Verification items for the finished model (mm, model axes). A direction names the side the tool comes from. Coordinates: 2 decimals unless noted, no trailing zeros. Loops run counter-clockwise (first coordinate to the right, second up) from the corner with the lowest first, then second, coordinate; pieces in that order, holes last.
Q1. Go/stop test with flat-tipped pins: P1, Ø0.6, axis at y = -6, z = -17, coming from the +X side; P2, Ø0.6, axis at x = -5, y = -4, coming from the +Z side; P3, Ø12, axis at x = -4.5, z = 2, coming from the -Y side. Record where each tip stops, or that it passes through.
Q2. Sectioned sample at C-C (x = -9.5). Enter the section's corners in (y, z).
Q3. Sectioned sample at A-A (z = 22). Enter the section's corners in (x, y), then the cut area to 3 significant figures.
Q4. Material ranges on probe 1 along Z at (x, y) = (0, -2.65); probe 2 along Z at (x, y) = (0, -3.95); probe 3 along Y at (x, z) = (-7.5, 17.5), recorded low to high.
Q5. Access from +Z, -Z, +X, -X, +Y, -Y to the whole of each face (thin tool, end or side, straight path). Record for faces 1 (the face through (3.374, -4.06, -1.503)), 2 (the face through (-8.597, -2.88, 27.073)).
Q6. Sectioned sample at B-B (z = -14). Enter the section's corners in (x, y), then the cut area to 3 significant figures.
Q7. Mould release check, pull along Z, two halves, no side actions. Record for faces 3 (the face through (0, -6.35, -15)), 4 (the face through (-9.165, -4.06, 5.715)), 5 (the face through (24.17, -2.88, 2.02)): +Z half, -Z half, draft (parallel to the pull), parting line (faces both ways), or undercut.
Q8. Sectioned sample at D-D (z = 14). Enter the section's corners in (x, y), then the cut area to 3 significant figures.
```python
from build123d import *

# Parameters (mm, degrees)
F0_R     = 1.182239
F0_R_2   = 0.817997
F1_DEPTH = 5.842
F2_DEPTH = 3.81
F3_DEPTH = 5.08
F4_DEPTH = 4.318
F5_R     = 1.71122
F6_DEPTH = 25.4
F7_DEPTH = 6.35


with BuildPart() as f1:
    # F0 (on Front) → F1 (new body)
    with BuildSketch(Plane.XZ):
        Polygon((-4.180855, -20.625193), (-4.353608, -20.920252), (-3.424949, -21.167446), (-3.28061, -20.625193), align=None)
        Polygon((3.424949, -21.167446), (4.353608, -20.920252), (4.180855, -20.625193), (3.28061, -20.625193), align=None)
        Polygon((22.26289, -6.835999), (22.26289, 1.657223), (4.394875, -5.754956), (2.197438, -5.957079), (0, -6.159202), (-2.197438, -5.957079), (-4.394875, -5.754956), (-22.26289, 1.657223), (-22.26289, -6.835999), (-22.832444, -9.118818), (-15.86828, -11.246894), (-14.217053, -15.145346), (-4.353608, -20.920252), (-4.180855, -20.625193), (-4.180855, -11.195441), (-3.601368, -9.465247), (0, -9.465247), (3.601368, -9.465247), (4.180855, -11.195441), (4.180855, -20.625193), (4.353608, -20.920252), (14.217053, -15.145346), (15.86828, -11.246894), (22.832444, -9.118818), align=None)
        Polygon((-15.86828, -11.246894), (-22.832444, -9.118818), (-22.26289, -10.434624), (-14.217053, -15.145346), align=None)
        Polygon((22.26289, -10.434624), (22.832444, -9.118818), (15.86828, -11.246894), (14.217053, -15.145346), align=None)
        Polygon((24.816887, 1.657223), (22.26289, 1.657223), (22.26289, -6.835999), (22.832444, -9.118818), (25.498668, -5.754956), align=None)
        with Locations((23.784082, -3.675047)):
            Circle(F0_R, mode=Mode.SUBTRACT)
        with Locations((23.597831, -0.42893)):
            Circle(F0_R_2, mode=Mode.SUBTRACT)
        Polygon((-22.26289, -6.835999), (-22.26289, 1.657223), (-24.816887, 1.657223), (-25.498668, -5.754956), (-22.832444, -9.118818), align=None)
        with Locations((-23.784082, -3.675047)):
            Circle(F0_R, mode=Mode.SUBTRACT)
        with Locations((-23.597831, -0.42893)):
            Circle(F0_R_2, mode=Mode.SUBTRACT)
        Polygon((-19.404403, 16.750786), (-22.26289, 15.816627), (-23.496922, 2.400486), (-22.26289, 1.657223), align=None)
        Polygon((23.496922, 2.400486), (22.26289, 15.816627), (19.404403, 16.750786), (22.26289, 1.657223), align=None)
        Polygon((24.816887, 1.657223), (23.496922, 2.400486), (22.26289, 1.657223), align=None)
        Polygon((-22.26289, 1.657223), (-23.496922, 2.400486), (-24.816887, 1.657223), align=None)
        Polygon((-19.404403, 16.750786), (-22.832444, 16.386179), (-22.26289, 15.816627), align=None)
        Polygon((22.26289, 15.816627), (22.832444, 16.386179), (19.404403, 16.750786), align=None)
        Polygon((22.832444, 16.386179), (22.136323, 20.879321), (5.009265, 22.700958), (2.695112, 21.684956), (0, 21.684956), (-2.695112, 21.684956), (-5.009265, 22.700958), (-22.136323, 20.879321), (-22.832444, 16.386179), (-19.404403, 16.750786), (-5.009265, 18.281856), (-2.695112, 17.265854), (0, 17.265854), (2.695112, 17.265854), (5.009265, 18.281856), (19.404403, 16.750786), align=None)
        Polygon((3.467637, 26.608711), (0, 26.608711), (-3.467637, 26.608711), (-4.353608, 27.524108), (-12.96019, 26.608711), (-16.187659, 24.61306), (-16.630644, 23.537237), (-22.136323, 20.879321), (-5.009265, 22.700958), (-2.695112, 21.684956), (0, 21.684956), (2.695112, 21.684956), (5.009265, 22.700958), (22.136323, 20.879321), (16.630644, 23.537237), (16.187659, 24.61306), (12.96019, 26.608711), (4.353608, 27.524108), align=None)
    extrude(amount=F1_DEPTH)

    # F0 (on Front) → F2 (join)
    with BuildSketch(Plane.XZ):
        with Locations((23.784082, -3.675047)):
            Circle(F0_R)
        with Locations((23.597831, -0.42893)):
            Circle(F0_R_2)
        with Locations((-23.784082, -3.675047)):
            Circle(F0_R)
        with Locations((-23.597831, -0.42893)):
            Circle(F0_R_2)
        Polygon((22.26289, 1.657223), (19.404403, 16.750786), (18.012892, 15.012917), (13.572707, 15.012917), (11.013955, 13.131482), (5.896451, 13.131482), (4.394875, 15.088174), (0, 15.088174), (-4.394875, 15.088174), (-5.896451, 13.131482), (-11.013955, 13.131482), (-13.572707, 15.012917), (-18.012892, 15.012917), (-19.404403, 16.750786), (-22.26289, 1.657223), (-4.394875, -5.754956), (-2.197438, -5.957079), (-1.331172, -3.868833), (0, -3.868833), (1.331172, -3.868833), (2.197438, -5.957079), (4.394875, -5.754956), align=None)
        Polygon((-2.750259, 0), (-4.015016, -3.048861), (-11.364689, 0), (-11.364689, 3.272761), (-7.025312, 8.089235), (-4.015016, 8.089235), (-1.832551, 11.701591), (0, 11.701591), (1.832551, 11.701591), (4.015016, 8.089235), (7.025312, 8.089235), (11.364689, 3.272761), (11.364689, 0), (4.015016, -3.048861), (2.750259, 0), (0, 0), align=None, mode=Mode.SUBTRACT)
    extrude(amount=F2_DEPTH)

    # F0 (on Front) → F3 (join)
    with BuildSketch(Plane.XZ):
        Polygon((0, -6.159202), (2.197438, -5.957079), (1.331172, -3.868833), (0, -3.868833), (-1.331172, -3.868833), (-2.197438, -5.957079), align=None)
    extrude(amount=F3_DEPTH)

    # F0 (on Front) → F4 (join)
    with BuildSketch(Plane.XZ):
        Polygon((-11.364689, 0), (-4.015016, -3.048861), (-2.750259, 0), (0, 0), (2.750259, 0), (4.015016, -3.048861), (11.364689, 0), (11.364689, 3.272761), (7.025312, 8.089235), (4.015016, 8.089235), (1.832551, 11.701591), (0, 11.701591), (-1.832551, 11.701591), (-4.015016, 8.089235), (-7.025312, 8.089235), (-11.364689, 3.272761), align=None)
        Polygon((18.012892, 15.012917), (19.404403, 16.750786), (5.009265, 18.281856), (2.695112, 17.265854), (0, 17.265854), (-2.695112, 17.265854), (-5.009265, 18.281856), (-19.404403, 16.750786), (-18.012892, 15.012917), (-13.572707, 15.012917), (-11.013955, 13.131482), (-5.896451, 13.131482), (-4.394875, 15.088174), (0, 15.088174), (4.394875, 15.088174), (5.896451, 13.131482), (11.013955, 13.131482), (13.572707, 15.012917), align=None)
    extrude(amount=F4_DEPTH)

    # F5 (on face) → F6 (cut)
    with BuildSketch(Plane.XZ.offset(5.842)):
        with Locations((0, 22.658981)):
            Circle(F5_R)
    extrude(amount=-F6_DEPTH, mode=Mode.SUBTRACT)

    # F0 (on Front) → F7 (join)
    with BuildSketch(Plane.XZ):
        Polygon((3.28061, -20.625193), (4.180855, -20.625193), (4.180855, -11.195441), (3.601368, -9.465247), (0, -9.465247), (-3.601368, -9.465247), (-4.180855, -11.195441), (-4.180855, -20.625193), (-3.28061, -20.625193), (0, -20.625193), align=None)
    extrude(amount=F7_DEPTH)


solid = f1.part
```
Geometry check:
1. P1: stops at x = 11.48
1. P2: stops at z = 27.49
1. P3: stops at y = -4.32
2. outline: (-5.84, -17.91) - (0, -17.91) - (0, 26.98) - (-5.84, 26.98) - (-5.84, 17.8) - (-4.32, 17.8) - (-4.32, 13.13) - (-3.81, 13.13) - (-3.81, 5.34) - (-4.32, 5.34) - (-4.32, -0.77) - (-3.81, -0.77) - (-3.81, -3.64) - (-5.84, -3.64) - close
3. outline: (-19.81, -5.84) - (-1.58, -5.84) - (-1.58, 0) - (-19.81, 0) - close; (1.58, -5.84) - (19.81, -5.84) - (19.81, 0) - (1.58, 0) - close
3. area: 213 mm2
4. probe 1: z = -20.63 to 20.95, 24.37 to 26.61
4. probe 2: z = -20.63 to -3.87, 0 to 11.7, 15.09 to 20.95, 24.37 to 26.61
4. probe 3: y = -4.32 to 0
5. face 1: -Y
5. face 2: +Z, -X, +Y, -Y
6. outline: (-16.17, -5.84) - (-4.18, -5.84) - (-4.18, -6.35) - (4.18, -6.35) - (4.18, -5.84) - (16.17, -5.84) - (16.17, 0) - (-16.17, 0) - close
6. area: 193 mm2
7. face 3: draft
7. face 4: undercut
7. face 5: +Z half
8. outline: (-22.43, -5.84) - (-19.93, -5.84) - (-19.93, -3.81) - (-12.2, -3.81) - (-12.2, -4.32) - (-5.23, -4.32) - (-5.23, -3.81) - (5.23, -3.81) - (5.23, -4.32) - (12.2, -4.32) - (12.2, -3.81) - (19.93, -3.81) - (19.93, -5.84) - (22.43, -5.84) - (22.43, 0) - (-22.43, 0) - close
8. area: 188 mm2
